```python
from build123d import *

# Parameters (mm, degrees)
F0_R     = 15.755887
F1_DEPTH = 101.6
F2_R     = 21.017988
F3_DEPTH = 38.1
F4_R     = 14.073652
F5_DEPTH = 101.601


with BuildPart() as f1:
    # F0 (on Top) → F1 (new body)
    with BuildSketch(Plane.XY):
        Circle(F0_R)
    extrude(amount=-F1_DEPTH)

    # F2 (on Top) → F3 (join)
    with BuildSketch(Plane.XY):
        Circle(F2_R)
    extrude(amount=-F3_DEPTH)

    # F4 (on face) → F5 (cut, through all)
    with BuildSketch(Plane.XY):
        Circle(F4_R)
    extrude(amount=-F5_DEPTH, mode=Mode.SUBTRACT)


solid = f1.part
```
Could you check a few things on this model? Use its own coordinates, in mm. A direction names the side the tool comes from. Coordinates: 2 decimals unless noted, no trailing zeros. Order: outer loops, then holes, each group sorted by start corner. A loop starts at its lowest first (then second) coordinate and runs counter-clockwise, first axis right, second up. Notation, with made-up numbers: M -23,-9.75 L -4,-9.75 A25 ccw -4,24.25 Z; hole C 3,12 d5. An arc over 180 degrees is marked long. Use a Markdown table: item, result. Add a question column.
Q1. I'm going to push flat-ended pins straight in: pin 1 (4 mm diameter, centred on x = 4, z = -42.5, fed in from -Y); pin 2 (6 mm diameter, centred on y = -4.5, z = -62.5, fed in from -X); pin 3 (5 mm diameter, centred on x = -8, z = -53, fed in from +Y). Where does each tip first touch, or does it pass through?
Q2. I want a section at C-C on z = -27. List the corners of the cut face in (x, y) for me, then the cut area to 3 significant figures.
Q3. We'd pull the mould along Y, two halves only. Please class faces 3 (the flat face through (-6, 13, -101.6)), 4 (the cylindrical face through (-3.05, -13.74, -50.09)), 5 (the cylindrical face through (-4.556, -20.518, -18.783)): pulls with the +Y half, pulls with the -Y half, needs draft (parallel to the pull), parting line crosses it, or undercut.
Q4. I want a section at A-A on y = 0. List the corners of the cut face in (x, z) for me, then the cut area to 3 significant figures.
Q5. If I drill on L1, parallel to Y at x = 0, z = -76; L2, parallel to Y at x = 0, z = -38; L3, parallel to X at y = 11.5, z = -13, over which ranges is the centre line in solid material (lowest first)?
Q6. Which directions (+Z, -Z, +X, -X, +Y, -Y) give clear straight access to the entire face, cutting with the end or side of a thin tool? Please do faces 1 (the flat face through (4, -14, 0)), 2 (the flat face through (-8, -14, -38.1)).
Checked values:
| question | item | result |
|---|---|---|
| 1 | pin 1 | y = -15.63 |
| 1 | pin 2 | x = -15.68 |
| 1 | pin 3 | y = 14.76 |
| 2 | outline | C 0,0 d42.04; hole C 0,0 d28.15 |
| 2 | area | 766 mm² |
| 3 | face 3 | needs draft |
| 3 | face 4 | undercut |
| 3 | face 5 | parting line crosses it |
| 4 | outline | M -21.02,-38.1 L -15.76,-38.1 L -15.76,-101.6 L -14.07,-101.6 L -14.07,0 L -21.02,0 Z; M 14.07,-101.6 L 15.76,-101.6 L 15.76,-38.1 L 21.02,-38.1 L 21.02,0 L 14.07,0 Z |
| 4 | area | 743 mm² |
| 5 | L1 | -15.76 to -14.07, 14.07 to 15.76 |
| 5 | L2 | -21.02 to -14.07, 14.07 to 21.02 |
| 5 | L3 | -17.59 to -8.11, 8.11 to 17.59 |
| 6 | face 1 | +Z, +X, -X, +Y, -Y |
| 6 | face 2 | -Z |
